from build123d import *

# Parameters (mm, degrees)
F1_DEPTH = 12.7
F2_R     = 3.175
F3_DEPTH = 12.7


with BuildPart() as f1:
    # F0 (on Front) → F1 (new body)
    with BuildSketch(Plane.XZ):
        with BuildLine():
            ThreePointArc((-3.680107, 18.691156), (-0.001675, 19.05), (3.676821, 18.691803))
            Line((3.676821, 18.691803), (-0.001412, 23.835839))
            Line((-0.001412, 23.835839), (-3.680107, 18.691156))
        make_face()
        with BuildLine():
            ThreePointArc((-10.964323, 15.578386), (-7.749863, 17.40236), (-4.243698, 18.571309))
            Line((-4.243698, 18.571309), (-9.696199, 21.774548))
            Line((-9.696199, 21.774548), (-10.964323, 15.578386))
        make_face()
        with BuildLine():
            ThreePointArc((-16.352708, 9.771972), (-14.158029, 12.745694), (-11.430443, 15.239668))
            Line((-11.430443, 15.239668), (-17.714425, 15.94824))
            Line((-17.714425, 15.94824), (-16.352708, 9.771972))
        make_face()
        with BuildLine():
            ThreePointArc((-18.913561, 2.275895), (-18.118144, 5.885181), (-16.64076, 9.272949))
            Line((-16.64076, 9.272949), (-22.669666, 7.364337))
            Line((-22.669666, 7.364337), (-18.913561, 2.275895))
        make_face()
        with BuildLine():
            ThreePointArc((4.240433, 18.572055), (7.746803, 17.403722), (10.961584, 15.580313))
            Line((10.961584, 15.580313), (9.693619, 21.775697))
            Line((9.693619, 21.775697), (4.240433, 18.572055))
        make_face()
        with BuildLine():
            ThreePointArc((11.427763, 15.241677), (14.155788, 12.748182), (16.35099, 9.774847))
            Line((16.35099, 9.774847), (17.712536, 15.950339))
            Line((17.712536, 15.950339), (11.427763, 15.241677))
        make_face()
        with BuildLine():
            ThreePointArc((16.63913, 9.275875), (18.117109, 5.888366), (18.913161, 2.27922))
            Line((18.913161, 2.27922), (22.668794, 7.367022))
            Line((22.668794, 7.367022), (16.63913, 9.275875))
        make_face()
        with BuildLine():
            ThreePointArc((18.97344, 1.70619), (19.03085, 0.853953), (19.05, 0))
            ThreePointArc((19.05, 0), (18.837584, -2.836885), (18.205075, -5.610505))
            Line((18.205075, -5.610505), (23.705411, -2.490119))
            Line((23.705411, -2.490119), (18.97344, 1.70619))
        make_face()
        with BuildLine():
            Line((20.643148, -11.916697), (18.02707, -6.158511))
            ThreePointArc((18.02707, -6.158511), (16.498621, -9.52355), (14.349165, -12.530122))
            Line((14.349165, -12.530122), (20.643148, -11.916697))
        make_face()
        with BuildLine():
            Line((14.011497, -19.282769), (13.963655, -12.95835))
            ThreePointArc((13.963655, -12.95835), (11.198664, -15.410789), (8.012155, -17.283167))
            Line((8.012155, -17.283167), (14.011497, -19.282769))
        make_face()
        with BuildLine():
            ThreePointArc((18.205075, -5.610505), (18.837584, -2.836885), (19.05, 0))
            ThreePointArc((19.05, 0), (19.03085, 0.853953), (18.97344, 1.70619))
            ThreePointArc((18.97344, 1.70619), (18.945467, 1.992933), (18.913161, 2.27922))
            ThreePointArc((18.913161, 2.27922), (18.117109, 5.888366), (16.63913, 9.275875))
            ThreePointArc((16.63913, 9.275875), (16.496947, 9.52645), (16.35099, 9.774847))
            ThreePointArc((16.35099, 9.774847), (14.155788, 12.748182), (11.427763, 15.241677))
            ThreePointArc((11.427763, 15.241677), (11.195954, 15.412758), (10.961584, 15.580313))
            ThreePointArc((10.961584, 15.580313), (7.746803, 17.403722), (4.240433, 18.572055))
            ThreePointArc((4.240433, 18.572055), (3.95908, 18.63406), (3.676821, 18.691803))
            ThreePointArc((3.676821, 18.691803), (-0.001675, 19.05), (-3.680107, 18.691156))
            ThreePointArc((-3.680107, 18.691156), (-3.962356, 18.633364), (-4.243698, 18.571309))
            ThreePointArc((-4.243698, 18.571309), (-7.749863, 17.40236), (-10.964323, 15.578386))
            ThreePointArc((-10.964323, 15.578386), (-11.198664, 15.410789), (-11.430443, 15.239668))
            ThreePointArc((-11.430443, 15.239668), (-14.158029, 12.745694), (-16.352708, 9.771972))
            ThreePointArc((-16.352708, 9.771972), (-16.498621, 9.52355), (-16.64076, 9.272949))
            ThreePointArc((-16.64076, 9.272949), (-18.118144, 5.885181), (-18.913561, 2.275895))
            ThreePointArc((-18.913561, 2.275895), (-18.945817, 1.989602), (-18.973739, 1.702854))
            ThreePointArc((-18.973739, 1.702854), (-18.945467, -1.992933), (-18.204088, -5.613705))
            ThreePointArc((-18.204088, -5.613705), (-18.117109, -5.888366), (-18.025987, -6.161681))
            ThreePointArc((-18.025987, -6.161681), (-16.496947, -9.52645), (-14.346962, -12.532644))
            ThreePointArc((-14.346962, -12.532644), (-14.155788, -12.748182), (-13.961377, -12.960805))
            ThreePointArc((-13.961377, -12.960805), (-11.195954, -15.412758), (-8.009116, -17.284576))
            ThreePointArc((-8.009116, -17.284576), (-7.746803, -17.403722), (-7.482718, -17.518888))
            ThreePointArc((-7.482718, -17.518888), (-3.95908, -18.63406), (-0.286422, -19.047847))
            ThreePointArc((-0.286422, -19.047847), (0.001675, -19.05), (0.28977, -19.047796))
            ThreePointArc((0.28977, -19.047796), (3.962356, -18.633364), (7.485798, -17.517572))
            ThreePointArc((7.485798, -17.517572), (7.749863, -17.40236), (8.012155, -17.283167))
            ThreePointArc((8.012155, -17.283167), (11.198664, -15.410789), (13.963655, -12.95835))
            ThreePointArc((13.963655, -12.95835), (14.158029, -12.745694), (14.349165, -12.530122))
            ThreePointArc((14.349165, -12.530122), (16.498621, -9.52355), (18.02707, -6.158511))
            ThreePointArc((18.02707, -6.158511), (18.118144, -5.885181), (18.205075, -5.610505))
        make_face()
        with BuildLine():
            Line((4.957131, -23.314675), (7.485798, -17.517572))
            ThreePointArc((7.485798, -17.517572), (3.962356, -18.633364), (0.28977, -19.047796))
            Line((0.28977, -19.047796), (4.957131, -23.314675))
        make_face()
        with BuildLine():
            Line((-4.954369, -23.315262), (-0.286422, -19.047847))
            ThreePointArc((-0.286422, -19.047847), (-3.95908, -18.63406), (-7.482718, -17.518888))
            Line((-7.482718, -17.518888), (-4.954369, -23.315262))
        make_face()
        with BuildLine():
            Line((-14.009212, -19.284429), (-8.009116, -17.284576))
            ThreePointArc((-8.009116, -17.284576), (-11.195954, -15.412758), (-13.961377, -12.960805))
            Line((-13.961377, -12.960805), (-14.009212, -19.284429))
        make_face()
        with BuildLine():
            Line((-20.641736, -11.919142), (-14.346962, -12.532644))
            ThreePointArc((-14.346962, -12.532644), (-16.496947, -9.52645), (-18.025987, -6.161681))
            Line((-18.025987, -6.161681), (-20.641736, -11.919142))
        make_face()
        with BuildLine():
            Line((-23.705116, -2.492928), (-18.204088, -5.613705))
            ThreePointArc((-18.204088, -5.613705), (-18.945467, -1.992933), (-18.973739, 1.702854))
            Line((-18.973739, 1.702854), (-23.705116, -2.492928))
        make_face()
    extrude(amount=F1_DEPTH)

    # F2 (on face) → F3 (cut)
    with BuildSketch(Plane.XZ.offset(12.7)):
        Circle(F2_R)
    extrude(amount=-F3_DEPTH, mode=Mode.SUBTRACT)


solid = f1.part
Input: part model. Units: mm. Frame: model coordinates. A direction names the side the tool comes from. Coordinates: 2 decimals unless noted, no trailing zeros. Loops run counter-clockwise (first coordinate to the right, second up) from the corner with the lowest first, then second, coordinate; pieces in that order, holes last.
Q1. Material intervals for line 1 (X direction, y = -12, z = -20); line 2 (X direction, y = -4.75, z = 21); line 3 (Z direction, x = -9.5, y = -4), sorted ascending.
Q2. Contact query for flat-ended pins moving along their axis: pin 1 (5 mm diameter, centred on y = -2.5, z = 2.5, fed in from +X); pin 2 (1.5 mm diameter, centred on x = -2, y = -10, fed in from +Z). Output: stop coordinate, or through.
Q3. Cut plane A-A (z = 0). Output: boundary loops of the cut face in (x, y) (3 decimals), then the cut area to 3 significant figures.
Q4. Set-up query: faces 4 (the face through (20.92, -6.26, -4.07)), 5 (the face through (-20.82, -6.26, 4.86)), 6 (the face through (1.86, -6.26, 21.23)), 7 (the face through (6.204, -6.261, -20.457)). Return all of +Z, -Z, +X, -X, +Y, -Y with unobstructed straight access to the full face (end or side cutting, diameter ignored); none if empty.
Q5. Draft query along X for faces 1 (the face through (-17.54, -6.26, -12.22)), 2 (the face through (17.452, -6.261, -12.228)), 3 (the face through (-1.815, -6.261, 21.3)). Return one class per face: +X half, -X half, draft (parallel to the pull), parting line (faces both ways), or undercut.
Working result:
1. line 1: x = -6.4 to -1.33, 1.33 to 6.4
1. line 2: x = -9.85 to -8.38, -2.03 to 2.03, 8.37 to 9.85
1. line 3: z = -17.78 to 21.66
2. pin 1: stops at x = 20.92
2. pin 2: stops at z = 22.09
3. outline: (-20.894, -12.7) - (-3.175, -12.7) - (-3.175, 0) - (-20.894, 0) - close; (3.175, -12.7) - (20.897, -12.7) - (20.897, 0) - (3.175, 0) - close
3. area: 450 mm2
4. face 4: +X, +Y, -Y
4. face 5: -X, +Y, -Y
4. face 6: +Z, +Y, -Y
4. face 7: -Z, +Y, -Y
5. face 1: -X half
5. face 2: +X half
5. face 3: undercut
